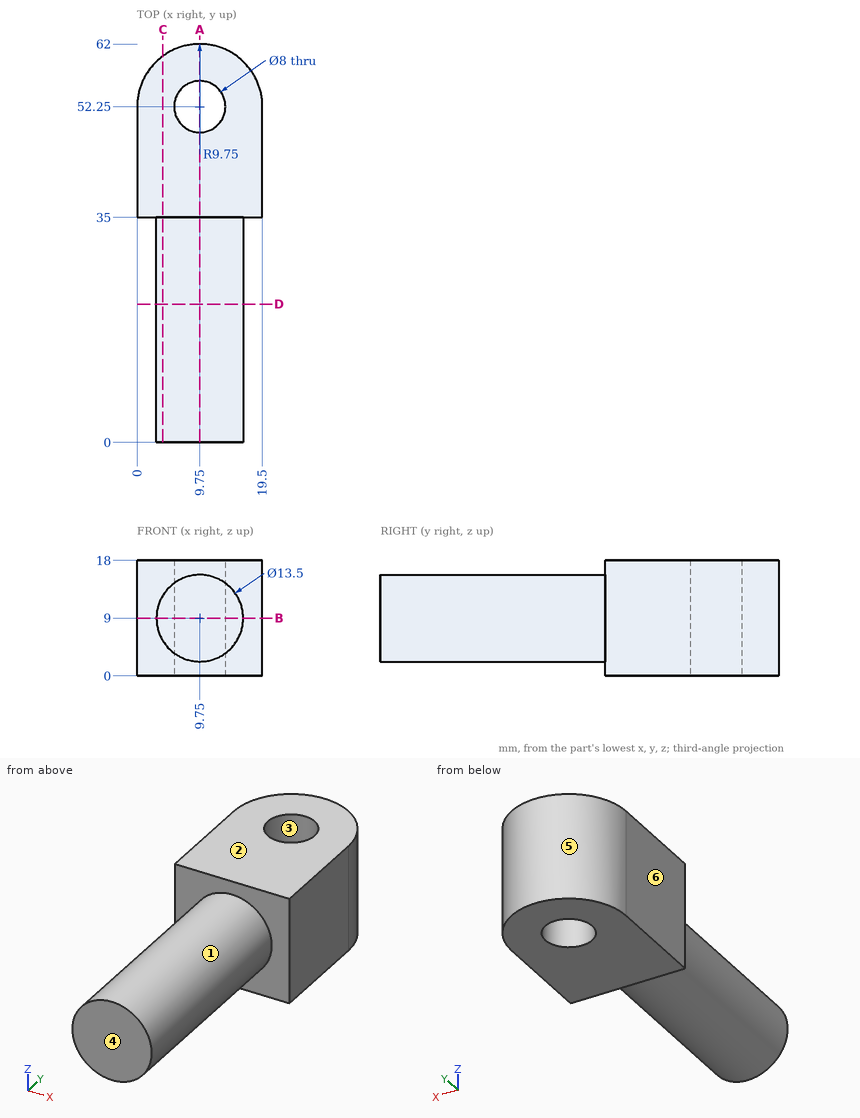
Answer from the drawing. Dimensions are ordinates in mm from the lowest x, y and z of the part. A direction names the side the tool comes from. Round coordinates to 2 decimals unless told otherwise and drop trailing zeros. Order: outer loops, then holes, each group sorted by start corner. A loop starts at its lowest first (then second) coordinate and runs counter-clockwise, first axis right, second up.
1) The part is cut by section D-D on y = 21.5. Write down the section's boundary in (x, z).
2) Straight lines are drawn through the part: L1, parallel to Y at x = 9.75, z = 5; L2, parallel to Y at x = 7.75, z = 13; L3, parallel to Y at x = 3, z = 1. For each, find the intervals that lie inside material, in ascending order.
3) For the marked faces 1 and 2, determine the directions among +Z, -Z, +X, -X, +Y, -Y from which every point of the face is accessible in a straight line to the end or side of a thin tool.
4) The part is cut by section B-B on z = 9. Write down the section's boundary in (x, y), plus the area to 3 significant figures.
5) The mould has two halves that part along Y. Classify the marked faces 3, 4, 5 and 6: released by +Y, released by -Y, zero draft, split by the parting line, or undercut.
6) Flat-ended cylindrical pins translate along their axes: pin 1 (1.5 mm diameter, centred on x = 4, y = 33, fed in from -Z); pin 2 (5 mm diameter, centred on x = 9.75, y = 52.25, fed in from -Z); pin 3 (10 mm diameter, centred on y = 23.5, z = 6.5, fed in from -X); pin 4 (6 mm diameter, centred on y = 30, z = 2, fed in from +X). Find the tip coordinate at first contact, or state that the pin passes through.
7) The part is cut by section C-C on x = 4. Write down the section's boundary in (y, z), plus the area to 3 significant figures.
8) The part is cut by section A-A on x = 9.75. Write down the section's boundary in (y, z).
Resolved:
1. outline: circle Ø13.5 at (9.75, 9)
2. L1: y = 0 to 48.25, 56.25 to 62
2. L2: y = 0 to 48.79, 55.71 to 61.79
2. L3: y = 35 to 59.29
3. face 1: -Y
3. face 2: +Z, +X, -X, +Y, -Y
4. outline: (0, 35) - (3, 35) - (3, 0) - (16.5, 0) - (16.5, 35) - (19.5, 35) - (19.5, 52.25) arc R9.75 ccw to (0, 52.25) - close; hole circle Ø8 at (9.75, 52.25)
4. area: 908 mm2
5. face 3: undercut
5. face 4: released by -Y
5. face 5: released by +Y
5. face 6: zero draft
6. pin 1: stops at z = 4.47
6. pin 2: passes through
6. pin 3: stops at x = 3
6. pin 4: stops at x = 15.19
7. outline: (0, 5.46) - (35, 5.46) - (35, 0) - (60.12, 0) - (60.12, 18) - (35, 18) - (35, 12.54) - (0, 12.54) - close
7. area: 700 mm2
8. outline: (0, 2.25) - (35, 2.25) - (35, 0) - (48.25, 0) - (48.25, 18) - (35, 18) - (35, 15.75) - (0, 15.75) - close; (56.25, 0) - (62, 0) - (62, 18) - (56.25, 18) - close
